Check sheet for the modelled part. Datum: model origin and axes. Units: mm. Face numbers are marked on the shaded views. A direction names the side the tool comes from. Round coordinates to 2 decimals unless told otherwise and drop trailing zeros. Write each loop counter-clockwise with the first axis right and the second up, starting at its lowest first coordinate (ties: lowest second). Pieces come first, ordered by that corner, then holes. Notation, with made-up numbers: M -40,-10.75 L 19,-10.75 A20 ccw 19,-2.75 Z; hole C 67.5,64 d7. An arc over 180 degrees is marked long. Put each result on its own line as item: value.
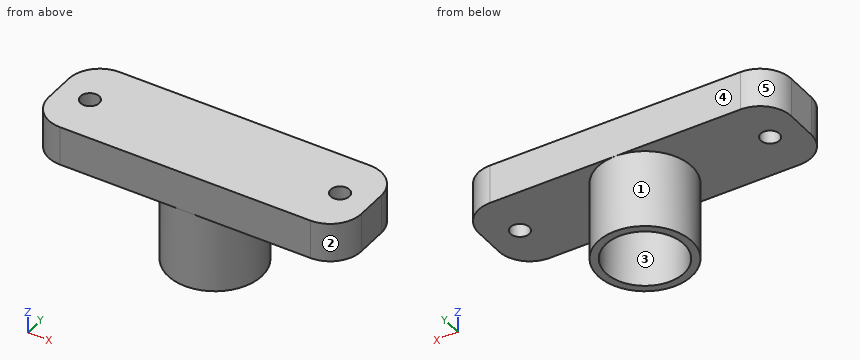
```python
from build123d import *

# Parameters (mm, degrees)
F0_W     = 25.4
F0_H     = 7.62
F1_DEPTH = 3.175
F2_R     = 2.54
F3_R     = 3.81
F3_R_2   = 3.175
F4_DEPTH = 6.35
F5_R     = 0.762
F6_DEPTH = 9.526


with BuildPart() as f1:
    # F0 (on Top) → F1 (new body)
    with BuildSketch(Plane.XY):
        Rectangle(F0_W, F0_H)
    extrude(amount=F1_DEPTH)

    # F2
    f2_edges = [f1.edges().sort_by_distance(p)[0] for p in [
        (-12.7, -3.81, 1.5875),
        (12.7, -3.81, 1.5875),
        (12.7, 3.81, 1.5875),
        (-12.7, 3.81, 1.5875),
    ]]
    fillet(f2_edges, radius=F2_R)

    # F3 (on face) → F4 (join)
    with BuildSketch(Plane(origin=(0, 0, 0), x_dir=(1, 0, 0), z_dir=(0, 0, -1))):
        Circle(F3_R)
        Circle(F3_R_2, mode=Mode.SUBTRACT)
    extrude(amount=F4_DEPTH)

    # F5 (on face) → F6 (cut, through all)
    with BuildSketch(Plane.XY.offset(3.175)):
        with Locations((-10.16, 0)):
            Circle(F5_R)
        with Locations((10.16, 0)):
            Circle(F5_R)
    extrude(amount=-F6_DEPTH, mode=Mode.SUBTRACT)


solid = f1.part
```
1. Cross-section at D-D (z = -4). Enter the section's corners in (x, y) (3 decimals).
Computed values:
outline: C 0,0 d7.62; hole C 0,0 d6.35
2. Cross-section at B-B (y = 0). Enter the section's corners in (x, z) (3 decimals).
Computed values:
outline: M -12.7,0 L -10.922,0 L -10.922,3.175 L -12.7,3.175 Z; M -9.398,0 L -3.81,0 L -3.81,-6.35 L -3.175,-6.35 L -3.175,0 L 3.175,0 L 3.175,-6.35 L 3.81,-6.35 L 3.81,0 L 9.398,0 L 9.398,3.175 L -9.398,3.175 Z; M 10.922,0 L 12.7,0 L 12.7,3.175 L 10.922,3.175 Z
3. Depth check by flat-ended pin: pin 1 Ø3 at (x, y) = (0.5, 1.5) entering from -Z; pin 2 Ø4 at (x, z) = (5.5, -3.5) entering from +Y; pin 3 Ø1.2 at (x, y) = (-10.16, 0) entering from +Z. Enter the tip coordinate at first touch or a pass-through.
Computed values:
pin 1: stops at z = 0
pin 2: stops at y = 1.51
pin 3: passes through
4. Access from +Z, -Z, +X, -X, +Y, -Y to the whole of each face (thin tool, end or side, straight path). Record for the marked faces 1 and 2.
Computed values:
face 1: -Z
face 2: +Z, -Z, +X, -Y
5. Cross-section at A-A (z = 1.75). Enter the section's corners in (x, y).
Computed values:
outline: M -12.7,-1.27 A2.54 ccw -10.16,-3.81 L 10.16,-3.81 A2.54 ccw 12.7,-1.27 L 12.7,1.27 A2.54 ccw 10.16,3.81 L -10.16,3.81 A2.54 ccw -12.7,1.27 Z; hole C -10.16,0 d1.52; hole C 10.16,0 d1.52
6. Cross-section at C-C (x = 7.5). Enter the section's corners in (y, z) (3 decimals).
Computed values:
outline: M -3.81,0 L 3.81,0 L 3.81,3.175 L -3.81,3.175 Z
7. Scan lines: probe 1 along X at (y, z) = (0, -2.5) (3 decimals); probe 2 along X at (y, z) = (-0.25, 2.5). Record each from-to range of solid material in increasing order.
Computed values:
probe 1: x = -3.81 to -3.175, 3.175 to 3.81
probe 2: x = -12.7 to -10.88, -9.44 to 9.44, 10.88 to 12.7
8. Release check for a two-part mould opening along X. For the marked faces 3, 4 and 5 record: +X half, -X half, draft (parallel to the pull), parting line (faces both ways), or undercut.
Computed values:
face 3: undercut
face 4: draft
face 5: -X half
